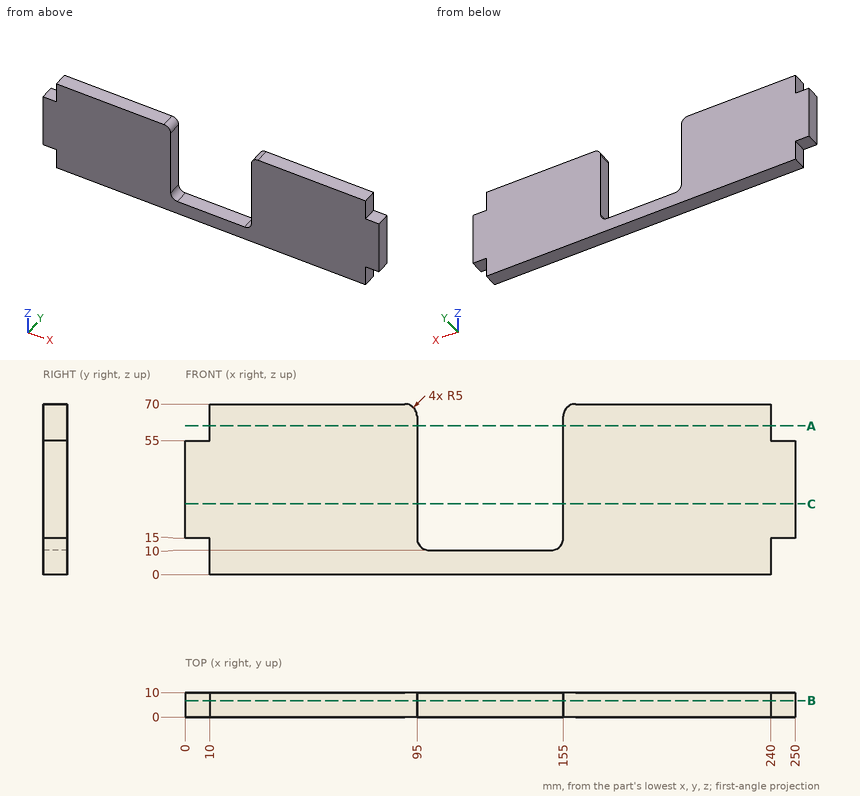
Geometry: see drawing. Coordinates: mm, zero at the bounding-box minimum. Round coordinates to 2 decimals unless told otherwise and drop trailing zeros. Loops run counter-clockwise (first coordinate to the right, second up) from the corner with the lowest first, then second, coordinate; pieces in that order, holes last. Notation, with made-up numbers: M 51.25,30.25 L 110.25,30.25 A19 cw 110.25,47.25 Z; hole C 24.25,-11.75 d8. An arc over 180 degrees is marked long. Use a Markdown table: item, result. Add a question column.
1. Ray query, line 1 along X through (y, z) = (2, 52); line 2 along X through (y, z) = (8, 14.5); line 3 along X through (y, z) = (4.5, 5). Return the intervals inside material, ascending. Write a range as [from, to].
2. Cut plane B-B, the plane y = 6.75. Output: boundary loops of the cut face in (x, z), and give its area (3 significant figures).
3. Cut plane A-A, the plane z = 61. Output: boundary loops of the cut face in (x, y).
4. Contact query for flat-ended pins moving along their axis: pin 1 (5 mm diameter, centred on x = 243, y = 6, fed in from -Z); pin 2 (3 mm diameter, centred on y = 6.5, z = 65.5, fed in from -X); pin 3 (3 mm diameter, centred on x = 243, y = 6.5, fed in from +Z). Output: stop coordinate, or through.
5. Cut plane C-C, the plane z = 29. Output: boundary loops of the cut face in (x, y).
Solution:
| question | item | result |
|---|---|---|
| 1 | line 1 | x = [0, 95], [155, 250] |
| 1 | line 2 | x = [10, 95.03], [154.97, 240] |
| 1 | line 3 | x = [10, 240] |
| 2 | outline | M 0,15 L 10,15 L 10,0 L 240,0 L 240,15 L 250,15 L 250,55 L 240,55 L 240,70 L 160,70 A5 ccw 155,65 L 155,15 A5 cw 150,10 L 100,10 A5 cw 95,15 L 95,65 A5 ccw 90,70 L 10,70 L 10,55 L 0,55 Z |
| 2 | area | 13,300 mm2 |
| 3 | outline | M 10,0 L 95,0 L 95,10 L 10,10 Z; M 155,0 L 240,0 L 240,10 L 155,10 Z |
| 4 | pin 1 | stops at z = 15 |
| 4 | pin 2 | stops at x = 10 |
| 4 | pin 3 | stops at z = 55 |
| 5 | outline | M 0,0 L 95,0 L 95,10 L 0,10 Z; M 155,0 L 250,0 L 250,10 L 155,10 Z |
